Verification items for the finished model (mm, model axes). Round coordinates to 2 decimals unless told otherwise and drop trailing zeros. Order: outer loops, then holes, each group sorted by start corner. A loop starts at its lowest first (then second) coordinate and runs counter-clockwise, first axis right, second up. Notation, with made-up numbers: M 16.5,32.5 L 31.5,32.5 A12 cw 31.5,36.5 Z; hole C 31.25,-15.75 d2. An arc over 180 degrees is marked long. Use CSV: the item, a comma, the result in double quotes. Start each with the question number.
Q1. Gauge pin test, flat ends, axial feed: pin 1 Ø1 at (x, z) = (99, 28.5) entering from -Y; pin 2 Ø1 at (x, y) = (65.5, 5) entering from -Z; pin 3 Ø2 at (x, z) = (0, 28) entering from +Y. Record the tip position at first contact, or that the pin passes through.
Q2. Sectioned sample at B-B (x = 63). Enter the section's corners in (y, z).
Q3. Scan lines: line 1 (X direction, y = 23, z = 28.95); line 2 (Z direction, x = 5, y = 27.5); line 3 (X direction, y = 22.5, z = 27.95) (3 decimals). Record each from-to range of solid material in increasing order.
Q4. Sectioned sample at A-A (y = 3.5). Enter the section's corners in (x, z).
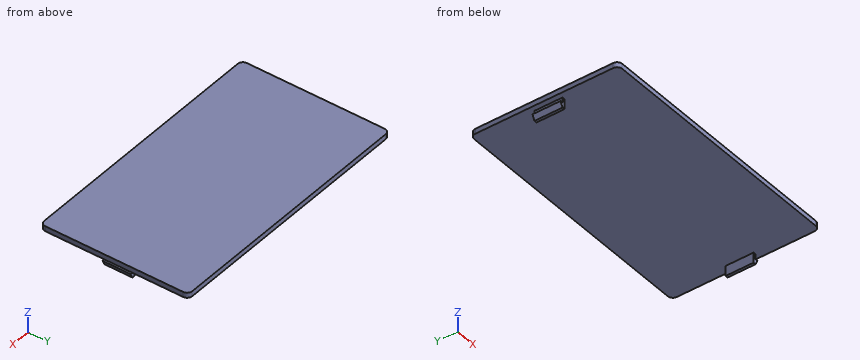
```python
from build123d import *

# Parameters (mm, degrees)
PAD002_DEPTH = 11
PAD001_DEPTH = 2


with BuildPart() as latches:
    # Sketch002 → Pad002 (new body)
    with BuildSketch(Plane.XZ):
        Polygon((1.5, 0), (1.5, -4), (0.5, -4), (-0.5, -2), (0.5, -2), (0.5, 0), (0.5, 0.5), (99.3, 0.5), (99.3, 0), (99.3, -2), (100.3, -2), (99.3, -4), (98.3, -4), (98.3, 0), align=None)
    extrude(amount=PAD002_DEPTH)


with BuildPart() as latches_1:
    # Body002 placement: moved
    add(latches.part.moved(Location((-0.4, 32.5, 0))))


with BuildPart() as obj1:
    # Sketch001 → Pad001 (new body)
    with BuildSketch(Plane.XY):
        with BuildLine():
            ThreePointArc((0, 56), (-1.414214, 55.414214), (-2, 54))
            Line((-2, 0), (-2, 54))
            ThreePointArc((-2, 0), (-1.414214, -1.414214), (0, -2))
            Line((99, -2), (0, -2))
            ThreePointArc((99, -2), (100.414214, -1.414214), (101, 0))
            Line((101, 54), (101, 0))
            ThreePointArc((101, 54), (100.414214, 55.414214), (99, 56))
            Line((0, 56), (99, 56))
        make_face()
    extrude(amount=PAD001_DEPTH)

    # Fusion002: union Latches
    add(latches_1.part)


with BuildPart() as obj1_1:
    # Fusion002 placement: moved
    add(obj1.part.moved(Location((0, 0, 30))))


solid = obj1_1.part
```
Verdict:
1,pin 1,"stops at y = 21.5"
1,pin 2,"stops at z = 30"
1,pin 3,"stops at y = 32.5"
2,outline,"M -2,30 L 56,30 L 56,32 L -2,32 Z"
3,line 1,"x = 0.1 to 1.1, 97.9 to 98.9"
3,line 2,"z = 30 to 32"
3,line 3,"x = -0.875 to 1.1, 97.9 to 99.875"
4,outline,"M -2,30 L 101,30 L 101,32 L -2,32 Z"
